Read the model definition and answer for the solid it produces. Units are mm, in the model's axes. Coordinates: 2 decimals unless noted, no trailing zeros. Loops run counter-clockwise (first coordinate to the right, second up) from the corner with the lowest first, then second, coordinate; pieces in that order, holes last.
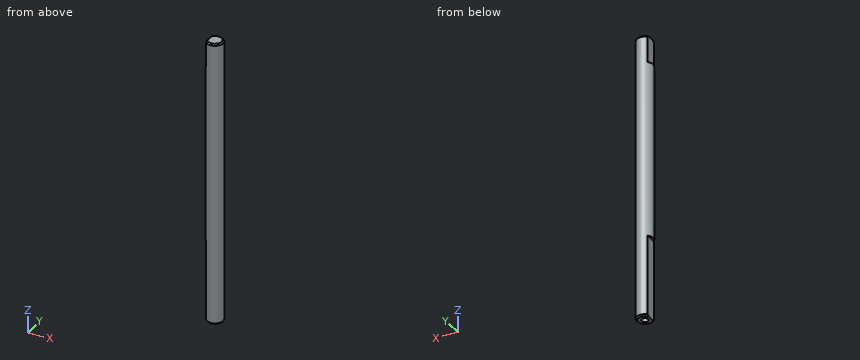
from build123d import *

# Parameters (mm, degrees)
SKETCH_1_R          = 3
EXTRUDE_1_DEPTH     = 105
CUT_EXTRUDE_1_DEPTH = 30
CUT_EXTRUDE_START   = -10
CUT_EXTRUDE_2_DEPTH = 10
M3X0_5_1_D          = 2.5
M3X0_5_1_DEPTH      = 10
M3X0_5_1_TIP        = 0.751075774
CHAMFER_1_SIZE      = 0.5


with BuildPart() as part:
    # 草图1 → 凸台-拉伸1 (new body)
    with BuildSketch(Plane.XY):
        Circle(SKETCH_1_R)
    extrude(amount=EXTRUDE_1_DEPTH)

    # 草图2 → 切除-拉伸1 (cut)
    with BuildSketch(Plane(origin=(0, 0, 0), x_dir=(-1, 0, 0), z_dir=(0, 0, -1))):
        with BuildLine():
            ThreePointArc((3, 0), (2.771638598, 1.148050297), (2.121320344, 2.121320344))
            Line((2.121320344, 2.121320344), (2.121320344, -2.121320344))
            ThreePointArc((2.121320344, -2.121320344), (2.771638598, -1.148050297), (3, 0))
        make_face()
    extrude(amount=-CUT_EXTRUDE_1_DEPTH, mode=Mode.SUBTRACT)

    # 草图3 → 切除-拉伸2 (cut)
    with BuildSketch(Plane.XY.offset(105).offset(CUT_EXTRUDE_START)):
        with BuildLine():
            Line((-2.121320344, -2.121320344), (-2.121320344, 2.121320344))
            ThreePointArc((-2.121320344, 2.121320344), (-3, 0), (-2.121320344, -2.121320344))
        make_face()
    extrude(amount=CUT_EXTRUDE_2_DEPTH, mode=Mode.SUBTRACT)

    # M3x0.5 螺纹孔1
    with Locations(Plane(origin=(0, 0, 0), x_dir=(-1, 0, 0), z_dir=(0, 0, -1))):
        with Locations((0, 0)):
            Hole(M3X0_5_1_D / 2, depth=M3X0_5_1_DEPTH)
            with Locations((0, 0, -(M3X0_5_1_DEPTH + M3X0_5_1_TIP / 2))):  # 118° drill point
                Cone(0, M3X0_5_1_D / 2, M3X0_5_1_TIP, mode=Mode.SUBTRACT)

    # 倒角1
    chamfer_1_edges = [part.edges().sort_by_distance(p)[0] for p in [
        (1.148050297, -2.771638598, 105),
        (1.148050297, 2.771638598, 0),
    ]]
    chamfer(chamfer_1_edges, length=CHAMFER_1_SIZE)


solid = part.part
Item 1: A cutting plane is placed at A-A on z = 58.5. Determine the outline of the cut face in (x, y).
Numbers:
outline: circle Ø6 at (0, 0)
Item 2: Given pin 1 (1.3 mm diameter, centred on y = -1, z = 19.5, fed in from -X); pin 2 (2 mm diameter, centred on x = 0, y = 0, fed in from -Z), each flat-ended and moving along its own axis, determine where each tip first touches the part or whether it passes through.
Numbers:
pin 1: stops at x = -2.12
pin 2: stops at z = 10.15
Item 3: Find the intervals of material crossed by line 1 along Y through (x, z) = (0, 7); line 2 along X through (y, z) = (0, 7.75); line 3 along Z through (x, y) = (-2.7, 1), in increasing order.
Numbers:
line 1: y = -3 to -1.25, 1.25 to 3
line 2: x = -2.12 to -1.25, 1.25 to 3
line 3: z = 30 to 95
